```python
from build123d import *

# Parameters (mm, degrees)
SKETCH1_R           = 11
SKETCH1_R_2         = 1.5
BOSS_EXTRUDE1_DEPTH = 2
FILLET2_R           = 5
FILLET1_R           = 2.5


with BuildPart() as part:
    # Sketch1 → Boss-Extrude1 (new body)
    with BuildSketch(Plane(origin=(0, 0, 0), x_dir=(1, 0, 0), z_dir=(0, 1, 0))):
        Polygon((21, 6), (28, 6), (28, -6), (21, -6), (21, -21), (-21, -21), (-21, -6), (-28, -6), (-28, 6), (-21, 6), (-21, 21), (-6, 21), (-6, 28), (6, 28), (6, 21), (21, 21), align=None)
        with Locations(Location((0, 0, 0), (0, 0, 270))):
            Circle(SKETCH1_R, mode=Mode.SUBTRACT)
        with Locations(Location((-25, 0, 0), (0, 0, 270))):
            Circle(SKETCH1_R_2, mode=Mode.SUBTRACT)
        with Locations(Location((0, 25, 0), (0, 0, 270))):
            Circle(SKETCH1_R_2, mode=Mode.SUBTRACT)
        with Locations(Location((25, 0, 0), (0, 0, 270))):
            Circle(SKETCH1_R_2, mode=Mode.SUBTRACT)
    extrude(amount=BOSS_EXTRUDE1_DEPTH)

    # Fillet2
    fillet2_edges = [part.edges().sort_by_distance(p)[0] for p in [
        (21, 1, 21),
        (-21, 1, 21),
        (-21, 1, -21),
        (21, 1, -21),
    ]]
    fillet(fillet2_edges, radius=FILLET2_R)

    # Fillet1
    fillet1_edges = [part.edges().sort_by_distance(p)[0] for p in [
        (28, 1, 6),
        (21, 1, 6),
        (-21, 1, 6),
        (-28, 1, 6),
        (-28, 1, -6),
        (-21, 1, -6),
        (-6, 1, -21),
        (-6, 1, -28),
        (6, 1, -28),
        (6, 1, -21),
        (21, 1, -6),
        (28, 1, -6),
    ]]
    fillet(fillet1_edges, radius=FILLET1_R)


solid = part.part
```
For this review, take the finished solid that the model builds, in its own axes (mm). A direction names the side the tool comes from. Give positions to 0.01 mm unless a question says otherwise; leave off trailing zeros. Loops run counter-clockwise (first coordinate to the right, second up) from the corner with the lowest first, then second, coordinate; pieces in that order, holes last. Notation, with made-up numbers: M 50.25,12 L 60.25,12 A30 ccw 60.25,37 Z; hole C -39.5,34 d3. An arc over 180 degrees is marked long. One line per item, written item: value. Start each with the question number.
Q1. Add section C-C (x = -9.5). Give the boundary of the cut face in (y, z), and give its area (3 significant figures).
Q2. Draft analysis for pull direction X (two halves, no side actions). For faces 4 (the face through (0.07, 0.99, -26.5)), 5 (the face through (24, 1, -6)), 6 (the face through (20, 1, -19)), 7 (the face through (-23.513, 0.986, -0.195)), state which applies: released by +X, released by -X, zero draft, split by the parting line, or undercut.
Q3. Add section D-D (z = -7.5). Give the boundary of the cut face in (x, y).
Q4. Machinability: for faces 1 (the face through (7, 0, -9)), 2 (the face through (-12, 1, -21)), 3 (the face through (21, 1, 12)), which of the approach directions +Z, -Z, +X, -X, +Y, -Y give a long, thin tool a straight path to every point of the face, cutting with its end or side? Answer none if there is none.
Q5. Add section A-A (x = 0). Give the boundary of the cut face in (y, z).
Q6. Add section B-B (z = 0). Give the boundary of the cut face in (x, y).
Q7. For L1, parallel to X at y = 1.4, z = 0; L2, parallel to Z at x = -1, y = 0.9; L3, parallel to Z at x = -0.5, y = 1.55, list the stretches that pass through material, from the lowest coordinate up.
Q8. Clearance check with flat-ended pins moving along their axes: pin 1 Ø0.6 at (y, z) = (1, -12.5) entering from +X; pin 2 Ø1 at (y, z) = (0.5, -11) entering from -X; pin 3 Ø2.5 at (x, z) = (0, -25) entering from +Y; pin 4 Ø1 at (x, y) = (12, 1) entering from -Z. State where each tip first meets the part, or that it passes through.
Reply:
1. outline: M 0,-21 L 2,-21 L 2,-5.55 L 0,-5.55 Z; M 0,5.55 L 2,5.55 L 2,21 L 0,21 Z
1. area: 61.8 mm²
2. face 4: undercut
2. face 5: zero draft
2. face 6: released by +X
2. face 7: undercut
3. outline: M -21.21,0 L -8.05,0 L -8.05,2 L -21.21,2 Z; M 8.05,0 L 21.21,0 L 21.21,2 L 8.05,2 Z
4. face 1: +Z, -Z, +X, -X, -Y
4. face 2: -Z, -X, +Y, -Y
4. face 3: +Z, +X, +Y, -Y
5. outline: M 0,-28 L 2,-28 L 2,-26.5 L 0,-26.5 Z; M 0,-23.5 L 2,-23.5 L 2,-11 L 0,-11 Z; M 0,11 L 2,11 L 2,21 L 0,21 Z
6. outline: M -28,0 L -26.5,0 L -26.5,2 L -28,2 Z; M -23.5,0 L -11,0 L -11,2 L -23.5,2 Z; M 11,0 L 23.5,0 L 23.5,2 L 11,2 Z; M 26.5,0 L 28,0 L 28,2 L 26.5,2 Z
7. L1: -28 to -26.5, -23.5 to -11, 11 to 23.5, 26.5 to 28
7. L2: -28 to -26.12, -23.88 to -10.95, 10.95 to 21
7. L3: -28 to -26.41, -23.59 to -10.99, 10.99 to 21
8. pin 1: x = 21
8. pin 2: x = -21
8. pin 3: through
8. pin 4: z = -21
